from build123d import *

# Parameters (mm, degrees)
SKETCH1_R                                      = 38.1
BOSS_EXTRUDE1_DEPTH                            = 6.35
CBORE_FOR_4_BUTTON_HEAD_CAP_SCREW1_D           = 2.8702
CBORE_FOR_4_BUTTON_HEAD_CAP_SCREW1_CBORE_D     = 4.826
CBORE_FOR_4_BUTTON_HEAD_CAP_SCREW1_CBORE_DEPTH = 1.905
CIRPATTERN1_COUNT                              = 8
SKETCH6_R                                      = 0.1984375
CUT_EXTRUDE1_DEPTH                             = 7.35
SKETCH7_R                                      = 0.396875
CIRPATTERN2_COUNT                              = 8


with BuildPart() as part:
    # Sketch1 → Boss-Extrude1 (new body)
    with BuildSketch(Plane(origin=(0, 0, 0), x_dir=(1, 0, 0), z_dir=(0, 1, 0))):
        Circle(SKETCH1_R)
    extrude(amount=BOSS_EXTRUDE1_DEPTH)

    # CBORE for #4 Button Head Cap Screw1 (through all)
    with Locations(Plane(origin=(0, 0, 0), x_dir=(-1, 0, 0), z_dir=(0, -1, 0))):
        with Locations((0, -33.3375)):
            cbore_for_4_button_head_cap_screw1 = CounterBoreHole(CBORE_FOR_4_BUTTON_HEAD_CAP_SCREW1_D / 2, CBORE_FOR_4_BUTTON_HEAD_CAP_SCREW1_CBORE_D / 2, CBORE_FOR_4_BUTTON_HEAD_CAP_SCREW1_CBORE_DEPTH)

    # CirPattern1: CBORE for #4 Button Head Cap Screw1 ×8 about axis
    cirpattern1_axis = Axis((0, 0, 0), (0, 1, 0))
    for i in range(1, CIRPATTERN1_COUNT):
        add(cbore_for_4_button_head_cap_screw1.rotate(cirpattern1_axis, i * 360 / CIRPATTERN1_COUNT), mode=Mode.SUBTRACT)

    # Sketch6 → Cut-Extrude1 (cut, through all)
    with BuildSketch(Plane(origin=(0, 6.35, 0), x_dir=(1, 0, 0), z_dir=(0, 1, 0))):
        with Locations((0, 9.525)):
            Circle(SKETCH6_R)
        with Locations((0, 11.049)):
            Circle(SKETCH6_R)
        with Locations((0, 12.573)):
            Circle(SKETCH6_R)
        with Locations((0, 14.097)):
            Circle(SKETCH6_R)
        with Locations((0, 15.621)):
            Circle(SKETCH6_R)
        with Locations((0, 17.145)):
            Circle(SKETCH6_R)
        with Locations((0, 18.669)):
            Circle(SKETCH6_R)
        with Locations((0, 20.193)):
            Circle(SKETCH6_R)
        with Locations((6.735192091, 6.735192091)):
            Circle(SKETCH6_R)
        with Locations((7.812822825, 7.812822825)):
            Circle(SKETCH6_R)
        with Locations((8.89045356, 8.89045356)):
            Circle(SKETCH6_R)
        with Locations((9.968084294, 9.968084294)):
            Circle(SKETCH6_R)
        with Locations((11.045715029, 11.045715029)):
            Circle(SKETCH6_R)
        with Locations((12.123345763, 12.123345763)):
            Circle(SKETCH6_R)
        with Locations((13.200976498, 13.200976498)):
            Circle(SKETCH6_R)
        with Locations((14.278607233, 14.278607233)):
            Circle(SKETCH6_R)
        with Locations((9.525, 0)):
            Circle(SKETCH6_R)
        with Locations((11.049, 0)):
            Circle(SKETCH6_R)
        with Locations((12.573, 0)):
            Circle(SKETCH6_R)
        with Locations((14.097, 0)):
            Circle(SKETCH6_R)
        with Locations((15.621, 0)):
            Circle(SKETCH6_R)
        with Locations((17.145, 0)):
            Circle(SKETCH6_R)
        with Locations((18.669, 0)):
            Circle(SKETCH6_R)
        with Locations((20.193, 0)):
            Circle(SKETCH6_R)
        with Locations((6.735192091, -6.735192091)):
            Circle(SKETCH6_R)
        with Locations((7.812822825, -7.812822825)):
            Circle(SKETCH6_R)
        with Locations((8.89045356, -8.89045356)):
            Circle(SKETCH6_R)
        with Locations((9.968084294, -9.968084294)):
            Circle(SKETCH6_R)
        with Locations((11.045715029, -11.045715029)):
            Circle(SKETCH6_R)
        with Locations((12.123345763, -12.123345763)):
            Circle(SKETCH6_R)
        with Locations((13.200976498, -13.200976498)):
            Circle(SKETCH6_R)
        with Locations((14.278607233, -14.278607232)):
            Circle(SKETCH6_R)
        with Locations((0, -9.525)):
            Circle(SKETCH6_R)
        with Locations((0, -11.049)):
            Circle(SKETCH6_R)
        with Locations((0, -12.573)):
            Circle(SKETCH6_R)
        with Locations((0, -14.097)):
            Circle(SKETCH6_R)
        with Locations((0, -15.621)):
            Circle(SKETCH6_R)
        with Locations((0, -17.145)):
            Circle(SKETCH6_R)
        with Locations((0, -18.669)):
            Circle(SKETCH6_R)
        with Locations((0, -20.193)):
            Circle(SKETCH6_R)
        with Locations((-6.735192091, -6.735192091)):
            Circle(SKETCH6_R)
        with Locations((-7.812822825, -7.812822825)):
            Circle(SKETCH6_R)
        with Locations((-8.89045356, -8.89045356)):
            Circle(SKETCH6_R)
        with Locations((-9.968084294, -9.968084294)):
            Circle(SKETCH6_R)
        with Locations((-11.045715029, -11.045715029)):
            Circle(SKETCH6_R)
        with Locations((-12.123345763, -12.123345763)):
            Circle(SKETCH6_R)
        with Locations((-13.200976498, -13.200976498)):
            Circle(SKETCH6_R)
        with Locations((-14.278607232, -14.278607233)):
            Circle(SKETCH6_R)
        with Locations((-9.525, 0)):
            Circle(SKETCH6_R)
        with Locations((-11.049, 0)):
            Circle(SKETCH6_R)
        with Locations((-12.573, 0)):
            Circle(SKETCH6_R)
        with Locations((-14.097, 0)):
            Circle(SKETCH6_R)
        with Locations((-15.621, 0)):
            Circle(SKETCH6_R)
        with Locations((-17.145, 0)):
            Circle(SKETCH6_R)
        with Locations((-18.669, 0)):
            Circle(SKETCH6_R)
        with Locations((-20.193, 0)):
            Circle(SKETCH6_R)
        with Locations((-6.735192091, 6.735192091)):
            Circle(SKETCH6_R)
        with Locations((-7.812822825, 7.812822825)):
            Circle(SKETCH6_R)
        with Locations((-8.89045356, 8.89045356)):
            Circle(SKETCH6_R)
        with Locations((-9.968084294, 9.968084294)):
            Circle(SKETCH6_R)
        with Locations((-11.045715029, 11.045715029)):
            Circle(SKETCH6_R)
        with Locations((-12.123345763, 12.123345763)):
            Circle(SKETCH6_R)
        with Locations((-13.200976498, 13.200976498)):
            Circle(SKETCH6_R)
        with Locations((-14.278607232, 14.278607232)):
            Circle(SKETCH6_R)
    extrude(amount=-CUT_EXTRUDE1_DEPTH, mode=Mode.SUBTRACT)

    # Cut-Sweep1: sweep along a curve in space
    with BuildLine() as cut_sweep1_path:
        Line((0, 6.35, -3.175), (0, 0, -4.7625))
    # Sketch7 → Cut-Sweep1 (sweep, cut)
    with BuildSketch(Plane(origin=(0, 6.35, 0), x_dir=(1, 0, 0), z_dir=(0, 1, 0))):
        with Locations((0, 3.175)):
            Circle(SKETCH7_R)
    cut_sweep1 = sweep(path=cut_sweep1_path.line, mode=Mode.SUBTRACT)

    # CirPattern2: Cut-Sweep1 ×8 about axis
    cirpattern2_axis = Axis((0, 6.35, 0), (0, 1, 0))
    for i in range(1, CIRPATTERN2_COUNT):
        add(cut_sweep1.rotate(cirpattern2_axis, i * 360 / CIRPATTERN2_COUNT), mode=Mode.SUBTRACT)


solid = part.part
The listing builds one solid part. Answer for the finished solid, in the listing's coordinates (mm). A direction names the side the tool comes from. Give positions to 0.01 mm unless a question says otherwise; leave off trailing zeros. Write each loop counter-clockwise with the first axis right and the second up, starting at its lowest first coordinate (ties: lowest second). Pieces come first, ordered by that corner, then holes. Notation, with made-up numbers: (-13, -0.5) - (4, -0.5) arc R24 ccw to (4, 25.5) - close; hole circle Ø9 at (-0.5, -9.5). An arc over 180 degrees is marked (long way). Use a Markdown table: item, result.
1. Each of these flat-tipped pins is pushed along its axis until it touches: P1, Ø2.5, axis at x = 0, z = -33, coming from the -Y side (3 decimals); P2, Ø1.5, axis at y = 5, z = 26.5, coming from the -X side; P3, Ø1, axis at y = 5, z = -1.5, coming from the +X side. Where does it stop, or does it pass through?
Values follow:
| item | result |
|---|---|
| P1 | stops at y = 1.905 |
| P2 | stops at x = -28.08 |
| P3 | stops at x = 38.09 |
2. A tool of negligible diameter and unlimited length cuts with its end or side. For faces 1 (the flat face through (-1, 0, -1)), 2 (the flat face through (25, 1.905, -22)), from which of +Z, -Z, +X, -X, +Y, -Y can it reach the whole face along a straight path? Write none if from no direction.
Values follow:
| item | result |
|---|---|
| face 1 | +Z, -Z, +X, -X, -Y |
| face 2 | -Y |
3. Section B-B on y = 3.5 is taken. Count the separate pieces of the cut face and the enclosed holes in it, plus the area to 3 significant figures.
Values follow:
| item | result |
|---|---|
| separate pieces | 1 |
| enclosed holes | 80 |
| area | 4,500 mm² |
4. Find the intervals of material crossed by probe 1 along Z at (x, y) = (23.5, 1.5); probe 2 along Z at (x, y) = (-33, 1); probe 3 along X at (y, z) = (0.5, 15.5), in increasing order. Write a range as from..to.
Values follow:
| item | result |
|---|---|
| probe 1 | z = -29.99..-25.99, -21.16..21.16, 25.99..29.99 |
| probe 2 | z = -19.04..-2.39, 2.39..19.04 |
| probe 3 | x = -34.8..-0.16, 0.16..34.8 |
5. Section A-A on x = 28 is taken. Write down the section's boundary in (y, z).
Values follow:
| item | result |
|---|---|
| outline | (0, -25.84) - (6.35, -25.84) - (6.35, 25.84) - (0, 25.84) - close |
